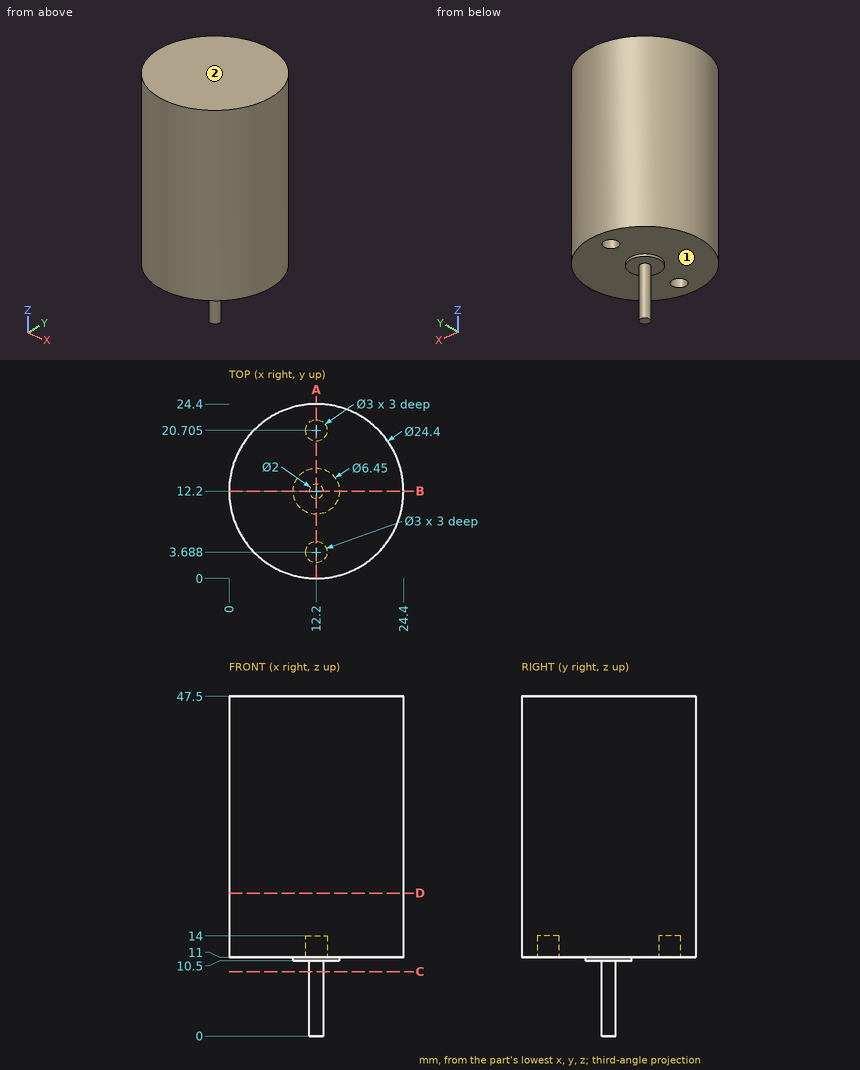
Part print with two shaded views. Sizes in mm from the minimum x, y, z corner. A direction names the side the tool comes from. Round coordinates to 2 decimals unless told otherwise and drop trailing zeros. Order: outer loops, then holes, each group sorted by start corner. A loop starts at its lowest first (then second) coordinate and runs counter-clockwise, first axis right, second up. Notation, with made-up numbers: M 31,86 L 68,86 A20 cw 68,111 Z; hole C 81,54.5 d7. An arc over 180 degrees is marked long. Put each result on its own line as item: value. Start each with the question number.
1. Drop flat-ended pins along their axis: pin 1 (2.5 mm diameter, centred on x = 12.5, y = 20.5, fed in from -Z); pin 2 (5 mm diameter, centred on y = 5.5, z = 17.5, fed in from -X) (1 decimal); pin 3 (2 mm diameter, centred on y = 4, z = 39.5, fed in from -X). Give the stop position or say it passes through.
2. Slice it at C-C on z = 9. List the corners of the cut face in (x, y).
3. Slice it at B-B on y = 12.2. List the corners of the cut face in (x, z) (1 decimal), then the cut area to 3 significant figures.
4. Slice it at D-D on z = 20. List the corners of the cut face in (x, y).
5. Tool access for the marked faces 1 and 2: list every direction of +Z, -Z, +X, -X, +Y, -Y with a clear straight run to the whole face (end or side of a thin tool).
6. Slice it at A-A on x = 12.2. List the corners of the cut face in (y, z) (1 decimal).
7. Drill centre lines: probe 1 along Y at (x, z) = (12.2, 12.45) (1 decimal); probe 2 along Z at (x, y) = (11, 21.5); probe 3 along Z at (x, y) = (20.75, 8.75). Where is each one in solid material? Low to high. Write a range as [from, to].
Findings:
1. pin 1: z = 11
1. pin 2: x = 0.7
1. pin 3: x = 2.35
2. outline: C 12.2,12.2 d2
3. outline: M 0,11 L 9,11 L 9,10.5 L 11.2,10.5 L 11.2,0 L 13.2,0 L 13.2,10.5 L 15.4,10.5 L 15.4,11 L 24.4,11 L 24.4,47.5 L 0,47.5 Z
3. area: 915 mm2
4. outline: C 12.2,12.2 d24.4
5. face 1: -Z
5. face 2: +Z, +X, -X, +Y, -Y
6. outline: M 0,11 L 2.2,11 L 2.2,14 L 5.2,14 L 5.2,11 L 9,11 L 9,10.5 L 11.2,10.5 L 11.2,0 L 13.2,0 L 13.2,10.5 L 15.4,10.5 L 15.4,11 L 19.2,11 L 19.2,14 L 22.2,14 L 22.2,11 L 24.4,11 L 24.4,47.5 L 0,47.5 Z
7. probe 1: [0, 2.2], [5.2, 19.2], [22.2, 24.4]
7. probe 2: [14, 47.5]
7. probe 3: [11, 47.5]
